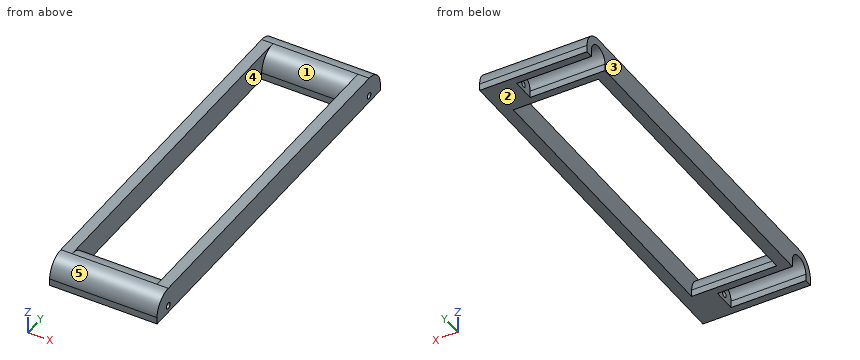
Autodesk Inventor part; units mm, degrees
ref_plane "YZ Plane" through (0, 0, 0) normal (1, 0, 0) x (0, 1, 0)
ref_plane "XZ Plane" through (0, 0, 0) normal (0, 1, 0) x (-1, 0, 0)
ref_plane "XY Plane" through (0, 0, 0) normal (0, 0, 1) x (1, 0, 0)
sketch "スケッチ1" plane through (0, 0, 0) normal (0, 0, 1) x (1, 0, 0)
  line L0 (-1.1, 1.1) -> (-1.1, 157.58) construction
  line L1 (42.18, 0) -> (0, 0) construction
  line L2 (43.28, 157.58) -> (43.28, 1.1) construction
  line L3 (0, 158.68) -> (42.18, 158.68) construction
  line L4 (43.28, 0) -> (-1.1, 0)
  line L5 (-1.1, 0) -> (-1.1, 158.68)
  line L6 (-1.1, 158.68) -> (43.28, 158.68)
  line L7 (43.28, 158.68) -> (43.28, 0)
  line L8 (49.121, 378.1158) -> (49.121, -108.9393) construction
  line L9 (49.121, -20) -> (-6.941, -20)
  line L10 (-6.941, -20) -> (-6.941, 178.68)
  line L11 (-6.941, 178.68) -> (49.121, 178.68)
  line L12 (49.121, 178.68) -> (49.121, -20)
  dimension "d0" = 20
  dimension "d1" = 20
  dimension "d2" = 5.841
  dimension "d15" = 5.841
extrude "押し出し1" add sketch "スケッチ1" along normal blind 13.64
sketch "スケッチ2" plane through (-6.941, -20, 0) normal (-1, 0, 0) x (0, 0, 1)
  circle A0 centre (3.64, 10) radius 1.6
  circle A1 centre (3.64, 188.68) radius 1.6
  point P0 (0, 20)
extrude "押し出し2" cut sketch "スケッチ2" against normal through all
fillet "フィレット1" radius 10 2 edges at (21.09, 178.68, 13.64) (21.09, -20, 13.64)
sketch "スケッチ3" plane through (-6.941, -20, 0) normal (-1, 0, 0) x (0, 0, 1)
  circle A0 centre (3.64, 188.68) radius 1.6 construction
  circle A1 centre (3.64, 10) radius 1.6 construction
  circle A2 centre (3.64, 188.68) radius 1.6
  circle A3 centre (3.64, 188.68) radius 6
  circle A4 centre (3.64, 10) radius 6
  point P0 (0, 20)
  dimension "d8" = 12
extrude "押し出し3" cut sketch "スケッチ3" against normal blind 39.062
fillet "フィレット2" [suppressed]
fillet "フィレット3" radius 10 2 edges at (21.09, 0, 13.64) (21.09, 158.68, 13.64)
sketch "スケッチ4" plane through (-6.941, -10, 13.64) normal (-1, 0, 0) x (0, 0, 1)
  line L0 (-13.64, -4.7697) -> (-13.64, -10)
  line L1 (-13.64, 173.9103) -> (-13.64, 4.7697)
  arc A0 (-13.64, -4.7697) -> (-13.64, 4.7697) centre (-10, 0) ccw
  line L2 (-13.64, 188.68) -> (-13.64, 183.4497)
  arc A1 (-13.64, 173.9103) -> (-13.64, 183.4497) centre (-10, 178.68) ccw
  line L3 (-10, -6) -> (-13.64, -6)
  line L4 (-10, 6) -> (-13.64, 6)
  line L5 (-10, 172.68) -> (-13.64, 172.68)
  line L6 (-10, 184.68) -> (-13.64, 184.68)
  point P0 (-13.64, 10)
extrude "押し出し4" cut sketch "スケッチ4" against normal up to surface (39.062 mm away)
equation "\"d1\" = d0"
equation "\"d2\" = d15"
properties part number "io_fix"
Can you work these out from the model? Positions are in its coordinate system, mm. Face numbers are marked on the shaded views. A direction names the side the tool comes from. Coordinates: 2 decimals unless noted, no trailing zeros. Write each loop counter-clockwise with the first axis right and the second up, starting at its lowest first coordinate (ties: lowest second). Pieces come first, ordered by that corner, then holes. Notation, with made-up numbers: (78, -18) -> (130, -18) arc R32 ccw to (130, 8) -> close; hole circle Ø5 at (16.25, -0.5). An arc over 180 degrees is marked (long way). Write each question's results on one line, items separated by ' | '. Start each with the question number.
Q1. If I drill on probe 1 along Y at (x, z) = (28, 2.5); probe 2 along Y at (x, z) = (42.25, 3.64); probe 3 along X at (y, z) = (46, 1.75), over which ranges is the centre line in solid material (lowest first)?
Q2. I'm going to push a flat-ended pin straight in: pin 1 (6 mm diameter, centred on x = 1, z = 10, fed in from +Y). Where does the tip first touch, or does it pass through?
Q3. Imagine slicing it at A-A (x = 35.5). State how many separate pieces and enclosed holes the cut face has, then the cut area to 3 significant figures.
Q4. On a 3-axis mill with a long thin cutter (end or side, diameter ignored), from which of +Z, -Z, +X, -X, +Y, -Y can I reach the whole of each face in a straight line? I mean the marked faces 1 and 2. Say none if no direction works.
Q5. Imagine slicing it at B-B (y = 63). Write out the boundary of the cut face in (x, z).
Q6. Imagine slicing it at D-D (z = 7). Write out the boundary of the cut face in (x, y).
Q7. We'd pull the mould along X, two halves only. Please class the marked faces 3, 4 and 5: +X half, -X half, draft (parallel to the pull), parting line (faces both ways), or undercut.
Taken from the geometry:
1) probe 1: y = -20 to -16, -4 to 0, 158.68 to 162.68, 174.68 to 178.68 | probe 2: y = -20 to -11.6, -8.4 to 0, 158.68 to 167.08, 170.28 to 178.68 | probe 3: x = -6.94 to -1.1, 43.28 to 49.12
2) pin 1: stops at y = 178.1
3) separate pieces: 2 | enclosed holes: 2 | area: 444 mm^2
4) face 1: +Z | face 2: -Z, +X, -X, +Y, -Y
5) outline: (-6.94, 0) -> (-1.1, 0) -> (-1.1, 13.64) -> (-6.94, 13.64) -> close; (43.28, 0) -> (49.12, 0) -> (49.12, 13.64) -> (43.28, 13.64) -> close
6) outline: (-6.94, -19.42) -> (49.12, -19.42) -> (49.12, 178.1) -> (-6.94, 178.1) -> (-6.94, 173.65) -> (32.12, 173.65) -> (32.12, 163.71) -> (-6.94, 163.71) -> (-6.94, -5.03) -> (32.12, -5.03) -> (32.12, -14.97) -> (-6.94, -14.97) -> close; hole (-1.1, -0.58) -> (43.28, -0.58) -> (43.28, 159.26) -> (-1.1, 159.26) -> close
7) face 3: -X half | face 4: undercut | face 5: draft
